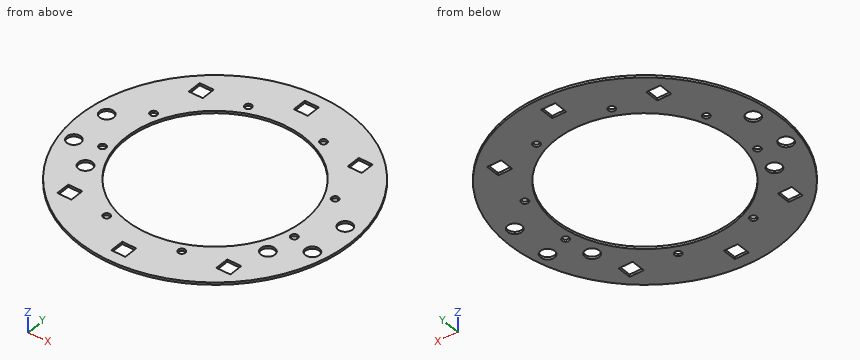
from build123d import *

# Parameters (mm, degrees)
CYLINDER531_R               = 3
CYLINDER531_DEPTH           = 7
CYLINDER530_R               = 3
CYLINDER530_DEPTH           = 7
CYLINDER445_R               = 1.5
CYLINDER445_DEPTH           = 100
CYLINDER445_PLACEMENT_ANGLE = 100
CYLINDER446_R               = 1.5
CYLINDER446_DEPTH           = 100
CYLINDER446_PLACEMENT_ANGLE = 135
CYLINDER447_R               = 1.5
CYLINDER447_DEPTH           = 100
CYLINDER448_R               = 1.5
CYLINDER448_DEPTH           = 100
CYLINDER448_PLACEMENT_ANGLE = 225
CYLINDER449_R               = 1.5
CYLINDER449_DEPTH           = 100
CYLINDER450_R               = 1.5
CYLINDER450_DEPTH           = 100
CYLINDER450_PLACEMENT_ANGLE = 55
CYLINDER451_R               = 1.5
CYLINDER451_DEPTH           = 100
CYLINDER444_R               = 1.5
CYLINDER444_DEPTH           = 100
CYLINDER444_PLACEMENT_ANGLE = 45
BOX154_W                    = 6
BOX154_H                    = 6
BOX154_DEPTH                = 10
BOX151_W                    = 6
BOX151_H                    = 6
BOX151_DEPTH                = 10
BOX155_W                    = 6
BOX155_H                    = 6
BOX155_DEPTH                = 10
BOX153_W                    = 6
BOX153_H                    = 6
BOX153_DEPTH                = 10
BOX156_W                    = 6
BOX156_H                    = 6
BOX156_DEPTH                = 10
BOX152_W                    = 6
BOX152_H                    = 6
BOX152_DEPTH                = 10
CYLINDER407_R               = 3
CYLINDER407_DEPTH           = 7
CYLINDER405_R               = 3
CYLINDER405_DEPTH           = 7
CYLINDER404_R               = 3
CYLINDER404_DEPTH           = 7
CYLINDER406_R               = 3
CYLINDER406_DEPTH           = 7
TUBE020_R                   = 58
TUBE020_R_2                 = 38
TUBE020_DEPTH               = 1


with BuildPart() as obj1:
    # Cylinder531 → Cylinder531 (new body)
    with BuildSketch(Plane(origin=(39, -21, 50), x_dir=(1, 0, 0), z_dir=(0, 0, 1))):
        Circle(CYLINDER531_R)
    extrude(amount=CYLINDER531_DEPTH)


with BuildPart() as compound337:
    # Cylinder530 → Cylinder530 (new body)
    with BuildSketch(Plane(origin=(-39, -21, 50), x_dir=(1, 0, 0), z_dir=(0, 0, 1))):
        Circle(CYLINDER530_R)
    extrude(amount=CYLINDER530_DEPTH)

    # Compound337: union obj1
    add(obj1.part)


with BuildPart() as compound337_1:
    # Compound337 placement: moved
    add(compound337.part.moved(Location((0, 0, -25))))


with BuildPart() as obj2:
    # Cylinder445 → Cylinder445 (new body)
    with BuildSketch(Plane.XY):
        Circle(CYLINDER445_R)
    extrude(amount=CYLINDER445_DEPTH)


with BuildPart() as obj2_1:
    # Cylinder445 placement: moved
    add(obj2.part.moved(Location((41.004432, -9.090464, 0))).rotate(Axis((41.004432, -9.090464, 0), (0, 0, 1)), CYLINDER445_PLACEMENT_ANGLE))


with BuildPart() as obj3:
    # Cylinder446 → Cylinder446 (new body)
    with BuildSketch(Plane.XY):
        Circle(CYLINDER446_R)
    extrude(amount=CYLINDER446_DEPTH)


with BuildPart() as obj3_1:
    # Cylinder446 placement: moved
    add(obj3.part.moved(Location((38.80294, 16.072704, 0))).rotate(Axis((38.80294, 16.072704, 0), (0, 0, 1)), CYLINDER446_PLACEMENT_ANGLE))


with BuildPart() as obj4:
    # Cylinder447 → Cylinder447 (new body)
    with BuildSketch(Plane(origin=(16.072704, 38.80294, 0), x_dir=(-1, 0, 0), z_dir=(0, 0, 1))):
        Circle(CYLINDER447_R)
    extrude(amount=CYLINDER447_DEPTH)


with BuildPart() as obj5:
    # Cylinder448 → Cylinder448 (new body)
    with BuildSketch(Plane.XY):
        Circle(CYLINDER448_R)
    extrude(amount=CYLINDER448_DEPTH)


with BuildPart() as obj5_1:
    # Cylinder448 placement: moved
    add(obj5.part.moved(Location((-16.072704, 38.80294, 0))).rotate(Axis((-16.072704, 38.80294, 0), (0, 0, 1)), CYLINDER448_PLACEMENT_ANGLE))


with BuildPart() as obj6:
    # Cylinder449 → Cylinder449 (new body)
    with BuildSketch(Plane(origin=(-38.80294, 16.072704, 0), x_dir=(0, -1, 0), z_dir=(0, 0, 1))):
        Circle(CYLINDER449_R)
    extrude(amount=CYLINDER449_DEPTH)


with BuildPart() as obj7:
    # Cylinder450 → Cylinder450 (new body)
    with BuildSketch(Plane.XY):
        Circle(CYLINDER450_R)
    extrude(amount=CYLINDER450_DEPTH)


with BuildPart() as obj7_1:
    # Cylinder450 placement: moved
    add(obj7.part.moved(Location((-41.004432, -9.090464, 0))).rotate(Axis((-41.004432, -9.090464, 0), (0, 0, -1)), CYLINDER450_PLACEMENT_ANGLE))


with BuildPart() as obj8:
    # Cylinder451 → Cylinder451 (new body)
    with BuildSketch(Plane(origin=(-16.072704, -38.80294, 0), x_dir=(1, 0, 0), z_dir=(0, 0, 1))):
        Circle(CYLINDER451_R)
    extrude(amount=CYLINDER451_DEPTH)


with BuildPart() as compound325:
    # Cylinder444 → Cylinder444 (new body)
    with BuildSketch(Plane.XY):
        Circle(CYLINDER444_R)
    extrude(amount=CYLINDER444_DEPTH)


with BuildPart() as compound325_1:
    # Cylinder444 placement: moved
    add(compound325.part.moved(Location((16.072704, -38.80294, 0))).rotate(Axis((16.072704, -38.80294, 0), (0, 0, 1)), CYLINDER444_PLACEMENT_ANGLE))

    # Compound325: union obj2, obj3, obj4, obj5, obj6, obj7, obj8
    add(obj2_1.part)
    add(obj3_1.part)
    add(obj4.part)
    add(obj5_1.part)
    add(obj6.part)
    add(obj7_1.part)
    add(obj8.part)


with BuildPart() as krychle154:
    # Box154 → Box154 (new body)
    with BuildSketch(Plane(origin=(-37, -39, 40), x_dir=(1, 0, 0), z_dir=(0, 0, 1))):
        with Locations((3, 3)):
            Rectangle(BOX154_W, BOX154_H)
    extrude(amount=BOX154_DEPTH)


with BuildPart() as krychle151:
    # Box151 → Box151 (new body)
    with BuildSketch(Plane(origin=(-3, -53, 40), x_dir=(1, 0, 0), z_dir=(0, 0, 1))):
        with Locations((3, 3)):
            Rectangle(BOX151_W, BOX151_H)
    extrude(amount=BOX151_DEPTH)


with BuildPart() as krychle155:
    # Box155 → Box155 (new body)
    with BuildSketch(Plane(origin=(31, 33, 40), x_dir=(1, 0, 0), z_dir=(0, 0, 1))):
        with Locations((3, 3)):
            Rectangle(BOX155_W, BOX155_H)
    extrude(amount=BOX155_DEPTH)


with BuildPart() as krychle153:
    # Box153 → Box153 (new body)
    with BuildSketch(Plane(origin=(-37, 33, 40), x_dir=(1, 0, 0), z_dir=(0, 0, 1))):
        with Locations((3, 3)):
            Rectangle(BOX153_W, BOX153_H)
    extrude(amount=BOX153_DEPTH)


with BuildPart() as krychle156:
    # Box156 → Box156 (new body)
    with BuildSketch(Plane(origin=(31, -39, 40), x_dir=(1, 0, 0), z_dir=(0, 0, 1))):
        with Locations((3, 3)):
            Rectangle(BOX156_W, BOX156_H)
    extrude(amount=BOX156_DEPTH)


with BuildPart() as compound316:
    # Box152 → Box152 (new body)
    with BuildSketch(Plane(origin=(-3, 47, 40), x_dir=(1, 0, 0), z_dir=(0, 0, 1))):
        with Locations((3, 3)):
            Rectangle(BOX152_W, BOX152_H)
    extrude(amount=BOX152_DEPTH)

    # Compound316: union Krychle154, Krychle151, Krychle155, Krychle153, Krychle156
    add(krychle154.part)
    add(krychle151.part)
    add(krychle155.part)
    add(krychle153.part)
    add(krychle156.part)


with BuildPart() as compound316_1:
    # Compound316 placement: moved
    add(compound316.part.moved(Location((0, 0, -18))))


with BuildPart() as obj9:
    # Cylinder407 → Cylinder407 (new body)
    with BuildSketch(Plane(origin=(51, -12, 50), x_dir=(1, 0, 0), z_dir=(0, 0, 1))):
        Circle(CYLINDER407_R)
    extrude(amount=CYLINDER407_DEPTH)


with BuildPart() as obj10:
    # Cylinder405 → Cylinder405 (new body)
    with BuildSketch(Plane(origin=(51, 6, 50), x_dir=(1, 0, 0), z_dir=(0, 0, 1))):
        Circle(CYLINDER405_R)
    extrude(amount=CYLINDER405_DEPTH)


with BuildPart() as obj11:
    # Cylinder404 → Cylinder404 (new body)
    with BuildSketch(Plane(origin=(-51, 6, 50), x_dir=(1, 0, 0), z_dir=(0, 0, 1))):
        Circle(CYLINDER404_R)
    extrude(amount=CYLINDER404_DEPTH)


with BuildPart() as compound312:
    # Cylinder406 → Cylinder406 (new body)
    with BuildSketch(Plane(origin=(-51, -12, 50), x_dir=(1, 0, 0), z_dir=(0, 0, 1))):
        Circle(CYLINDER406_R)
    extrude(amount=CYLINDER406_DEPTH)

    # Compound312: union obj9, obj10, obj11
    add(obj9.part)
    add(obj10.part)
    add(obj11.part)


with BuildPart() as compound312_1:
    # Compound312 placement: moved
    add(compound312.part.moved(Location((0, 0, -25))))


with BuildPart() as cut:
    # Tube020 → Tube020 (new body)
    with BuildSketch(Plane.XY.offset(31)):
        Circle(TUBE020_R)
        Circle(TUBE020_R_2, mode=Mode.SUBTRACT)
    extrude(amount=TUBE020_DEPTH)

    # Cut161: cut Compound312
    add(compound312_1.part, mode=Mode.SUBTRACT)

    # Cut163: cut Compound316
    add(compound316_1.part, mode=Mode.SUBTRACT)

    # Cut173: cut Compound325
    add(compound325_1.part, mode=Mode.SUBTRACT)

    # Cut: cut Compound337
    add(compound337_1.part, mode=Mode.SUBTRACT)


solid = cut.part
Work out the finished part from the listing and answer in its coordinate system (mm). Round coordinates to 2 decimals unless told otherwise and drop trailing zeros. Write each loop counter-clockwise with the first axis right and the second up, starting at its lowest first coordinate (ties: lowest second). Pieces come first, ordered by that corner, then holes.
1) A cutting plane is placed at A-A (y = 0). Give the vertices of the cut face in (x, z).
2) A cutting plane is placed at B-B (x = -51). Give the vertices of the cut face in (y, z).
3) A cutting plane is placed at D-D (x = 27). Give the vertices of the cut face in (y, z).
4) A cutting plane is placed at C-C (y = -21). Give the vertices of the cut face in (x, z).
5) Straight lines are drawn through the part: line 1 (Y direction, x = -0.5, z = 31.25); line 2 (Y direction, x = -39, z = 31.5); line 3 (X direction, y = -21, z = 31.2). For each, find the intervals that lie inside material, in ascending order.
Completed:
1. outline: (-58, 31) - (-38, 31) - (-38, 32) - (-58, 32) - close; (38, 31) - (58, 31) - (58, 32) - (38, 32) - close
2. outline: (-27.62, 31) - (-15, 31) - (-15, 32) - (-27.62, 32) - close; (-9, 31) - (3, 31) - (3, 32) - (-9, 32) - close; (9, 31) - (27.62, 31) - (27.62, 32) - (9, 32) - close
3. outline: (-51.33, 31) - (-26.74, 31) - (-26.74, 32) - (-51.33, 32) - close; (26.74, 31) - (51.33, 31) - (51.33, 32) - (26.74, 32) - close
4. outline: (-54.06, 31) - (-42, 31) - (-42, 32) - (-54.06, 32) - close; (-36, 31) - (-31.67, 31) - (-31.67, 32) - (-36, 32) - close; (31.67, 31) - (36, 31) - (36, 32) - (31.67, 32) - close; (42, 31) - (54.06, 31) - (54.06, 32) - (42, 32) - close
5. line 1: y = -58 to -53, -47 to -38, 38 to 47, 53 to 58
5. line 2: y = -42.93 to -24, -18 to 14.59, 17.56 to 42.93
5. line 3: x = -54.06 to -42, -36 to -31.67, 31.67 to 36, 42 to 54.06
